Job drawing, mm, ordinate dimensions from the low corner. One solid piece. A direction names the side the tool comes from. Round coordinates to 2 decimals unless told otherwise and drop trailing zeros. Loops run counter-clockwise (first coordinate to the right, second up) from the corner with the lowest first, then second, coordinate; pieces in that order, holes last. Notation, with made-up numbers: M 32,33 L 63,33 A20 cw 63,55 Z; hole C 49,83.25 d1. An arc over 180 degrees is marked long. Use a Markdown table: item, result. Add a question column.
(1) Band-saw the part on A-A, the plane y = 9.1. Write the cut outline in (x, z), and give its area (3 significant figures).
(2) Band-saw the part on C-C, the plane x = 5. Write the cut outline in (y, z), and give its area (3 significant figures).
(3) Two-plate mould, pull along X, no slides. Class the marked faces 4, 5 and 6: released by +X, released by -X, zero draft, split by the parting line, or undercut.
(4) Wall check: L1, parallel to X at y = 12.25, z = 34.5; L2, parallel to Y at x = 31, z = 51; L3, parallel to Z at x = 58, y = 7. Give the ranges that are in metal, low to high.
(5) Flat gauge pins, fed straight in: P1, Ø6.5, axis at y = 3.5, z = 38.5, coming from the +X side; P2, Ø1.6, axis at x = 77, y = 9.1, coming from the +Z side; P3, Ø1, axis at y = 9.5, z = 32, coming from the -X side; P4, Ø4, axis at x = 40, y = 7.5, coming from the -Z side. Where does each tip first touch, or does it go through?
(6) Band-saw the part on B-B, the plane z = 4. Write the cut outline in (x, y).
(7) Which spindle directions (+Z, -Z, +X, -X, +Y, -Y) get a long thin tool onto all of the face, cutting with end or side? Do the marked faces 1, 2 and 3. Say none if no direction does.
(8) Band-saw the part on D-D, the plane z = 41.5. Write the cut outline in (x, y), and give its area (3 significant figures).
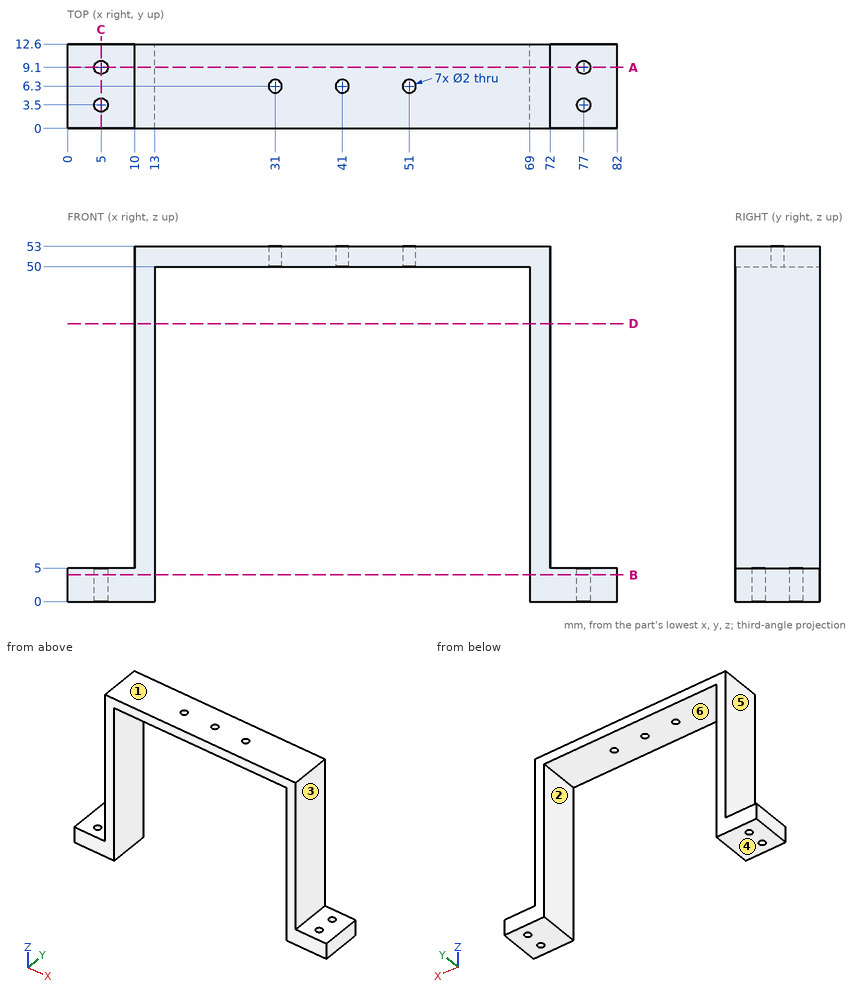
Return value:
| question | item | result |
|---|---|---|
| 1 | outline | M 0,0 L 4,0 L 4,5 L 0,5 Z; M 6,0 L 13,0 L 13,50 L 69,50 L 69,0 L 76,0 L 76,5 L 72,5 L 72,53 L 10,53 L 10,5 L 6,5 Z; M 78,0 L 82,0 L 82,5 L 78,5 Z |
| 1 | area | 566 mm^2 |
| 2 | outline | M 0,0 L 2.5,0 L 2.5,5 L 0,5 Z; M 4.5,0 L 8.1,0 L 8.1,5 L 4.5,5 Z; M 10.1,0 L 12.6,0 L 12.6,5 L 10.1,5 Z |
| 2 | area | 43.0 mm^2 |
| 3 | face 4 | zero draft |
| 3 | face 5 | released by -X |
| 3 | face 6 | undercut |
| 4 | L1 | 10 to 13, 69 to 72 |
| 4 | L2 | 0 to 5.3, 7.3 to 12.6 |
| 4 | L3 | 50 to 53 |
| 5 | P1 | x = 72 |
| 5 | P2 | through |
| 5 | P3 | x = 10 |
| 5 | P4 | z = 50 |
| 6 | outline | M 0,0 L 13,0 L 13,12.6 L 0,12.6 Z; M 69,0 L 82,0 L 82,12.6 L 69,12.6 Z; hole C 5,3.5 d2; hole C 5,9.1 d2; hole C 77,3.5 d2; hole C 77,9.1 d2 |
| 7 | face 1 | +Z, +X, -X, +Y, -Y |
| 7 | face 2 | -Z, +Y, -Y |
| 7 | face 3 | +Z, +X, +Y, -Y |
| 8 | outline | M 10,0 L 13,0 L 13,12.6 L 10,12.6 Z; M 69,0 L 72,0 L 72,12.6 L 69,12.6 Z |
| 8 | area | 75.6 mm^2 |
